Work out the finished part from the listing and answer in its coordinate system (mm). Face numbers are marked on the shaded views. Give positions to 0.01 mm unless a question says otherwise; leave off trailing zeros. Loops run counter-clockwise (first coordinate to the right, second up) from the corner with the lowest first, then second, coordinate; pieces in that order, holes last.
```python
from build123d import *

# Parameters (mm, degrees)
SKETCH2_R           = 17.416697508
BOSS_EXTRUDE1_DEPTH = 20
SKETCH7_R           = 17.416697508
CUT_EXTRUDE2_DEPTH  = 20
CIRPATTERN1_COUNT   = 6
SKETCH8_R           = 33.646475863
BOSS_EXTRUDE2_DEPTH = 30
SKETCH10_R          = 17.416697508
CUT_EXTRUDE3_DEPTH  = 30
CHAMFER1_SIZE2      = 3.639702343
CHAMFER1_SIZE       = 10


with BuildPart() as part:
    # Sketch2 → Boss-Extrude1 (new body)
    with BuildSketch(Plane.XY):
        with BuildLine():
            ThreePointArc((32.5, 121.291651246), (0, 163.646475863), (-32.5, 121.291651246))
            ThreePointArc((-32.5, 121.291651246), (-48.176762068, 83.444599647), (-88.791651246, 88.791651246))
            ThreePointArc((-88.791651246, 88.791651246), (-141.722005337, 81.823237932), (-121.291651246, 32.5))
            ThreePointArc((-121.291651246, 32.5), (-96.353524137, 0), (-121.291651246, -32.5))
            ThreePointArc((-121.291651246, -32.5), (-141.722005337, -81.823237932), (-88.791651246, -88.791651246))
            ThreePointArc((-88.791651246, -88.791651246), (-48.176762068, -83.444599647), (-32.5, -121.291651246))
            ThreePointArc((-32.5, -121.291651246), (0, -163.646475863), (32.5, -121.291651246))
            ThreePointArc((32.5, -121.291651246), (48.176762068, -83.444599647), (88.791651246, -88.791651246))
            ThreePointArc((88.791651246, -88.791651246), (141.722005337, -81.823237932), (121.291651246, -32.5))
            ThreePointArc((121.291651246, -32.5), (96.353524137, 0), (121.291651246, 32.5))
            ThreePointArc((121.291651246, 32.5), (141.722005337, 81.823237932), (88.791651246, 88.791651246))
            ThreePointArc((88.791651246, 88.791651246), (48.176762068, 83.444599647), (32.5, 121.291651246))
        make_face()
        with Locations((0, 130)):
            Circle(SKETCH2_R, mode=Mode.SUBTRACT)
        with Locations((112.583302492, 65)):
            Circle(SKETCH2_R, mode=Mode.SUBTRACT)
        with Locations((112.583302492, -65)):
            Circle(SKETCH2_R, mode=Mode.SUBTRACT)
        with Locations((0, -130)):
            Circle(SKETCH2_R, mode=Mode.SUBTRACT)
        with Locations((-112.583302492, -65)):
            Circle(SKETCH2_R, mode=Mode.SUBTRACT)
        with Locations((-112.583302492, 65)):
            Circle(SKETCH2_R, mode=Mode.SUBTRACT)
    extrude(amount=BOSS_EXTRUDE1_DEPTH)

    # Sketch4 → Revolve1 (revolve)
    with BuildSketch(Plane(origin=(0, 0, 0), x_dir=(0, 0, -1), z_dir=(1, 0, 0)), mode=Mode.PRIVATE) as revolve1_sk:
        Polygon((-20, 163.646475863), (-30, 158.646475863), (-30, 153.646475863), (-20, 153.646475863), align=None)
    revolve1 = revolve(revolve1_sk.sketch.rotate(Axis((0, 130, 0), (0, 0, 1)), 90), axis=Axis((0, 130, 0), (0, 0, 1)))

    # Sketch7 → Cut-Extrude2 (cut)
    with BuildSketch(Plane.XY):
        Circle(SKETCH7_R)
    extrude(amount=CUT_EXTRUDE2_DEPTH, mode=Mode.SUBTRACT)

    # CirPattern1: Revolve1 ×6 about axis
    cirpattern1_axis = Axis((0, 0, 0), (0, 0, 1))
    for i in range(1, CIRPATTERN1_COUNT):
        add(revolve1.rotate(cirpattern1_axis, i * 360 / CIRPATTERN1_COUNT))

    # Sketch8 → Boss-Extrude2 (add)
    with BuildSketch(Plane.XY):
        Circle(SKETCH8_R)
    extrude(amount=BOSS_EXTRUDE2_DEPTH)

    # Sketch10 → Cut-Extrude3 (cut)
    with BuildSketch(Plane.XY):
        Circle(SKETCH10_R)
    extrude(amount=CUT_EXTRUDE3_DEPTH, mode=Mode.SUBTRACT)

    # Chamfer1
    chamfer1_edges = [part.edges().sort_by_distance(p)[0] for p in [
        (-33.646475863, 0, 30),
    ]]
    chamfer1_side = [part.faces().sort_by_distance(p)[0] for p in [
        (-33.646475863, 0, 29.927205953),
    ]]
    chamfer(chamfer1_edges, length=CHAMFER1_SIZE - 0.0001, length2=CHAMFER1_SIZE2 - 0.0001, reference=chamfer1_side[0])  # a hair under: the kernel refuses the full size


solid = part.part
```
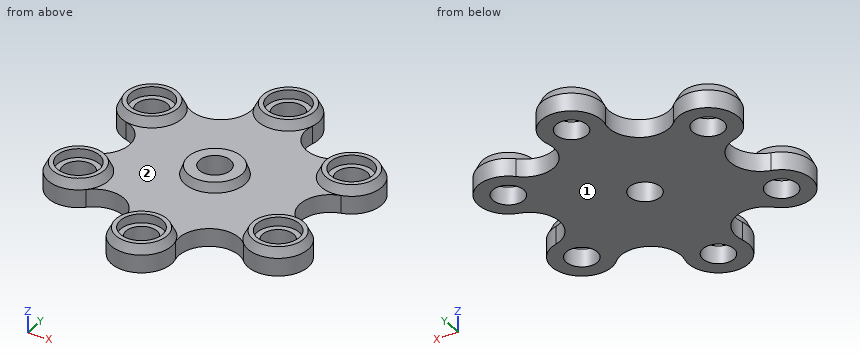
Q1. Section A-A on y = -130 is taken. Give the vertices of the cut face in (x, z).
Q2. Section D-D on x = 0 is taken. State how many separate pieces and enclosed holes the cut face has, plus the area to 3 significant figures.
Q3. Given pin 1 (10 mm diameter, centred on x = -0.5, z = 26, fed in from -Y); pin 2 (2 mm diameter, centred on x = -17.5, y = 58.5, fed in from +Z); pin 3 (12 mm diameter, centred on y = 83, z = 4, fed in from -X); pin 4 (23.5 mm diameter, centred on x = -2.5, y = 131, fed in from +Z), each flat-ended and moving along its own axis, determine where each tip first touches the part or whether it passes through.
Q4. Consider line 1 along Y through (x, z) = (110, 18.25); line 2 along Y through (x, z) = (-121.5, 27.75); line 3 along Y through (x, z) = (65, 17). Determine where each line is inside the solid, lowest interval first.
Q5. Section B-B on z = 8.5 is taken. Give the vertices of the cut face in (x, y).
Q6. Determine the mould class of the marked faces 1 and 2 for opening direction X: +X half, -X half, draft (parallel to the pull), parting line (faces both ways), or undercut.
Q7. Section C-C on y = 65 is taken. Give the vertices of the cut face in (x, z), plus the area to 3 significant figures.
Check result:
1. outline: (-33.65, 0) - (-17.42, 0) - (-17.42, 20) - (-23.65, 20) - (-23.65, 30) - (-28.65, 30) - (-33.65, 20) - close; (17.42, 0) - (33.65, 0) - (33.65, 20) - (28.65, 30) - (23.65, 30) - (23.65, 20) - (17.42, 20) - close
2. separate pieces: 4
2. enclosed holes: 0
2. area: 5,040 mm2
3. pin 1: stops at y = -163.14
3. pin 2: stops at z = 20
3. pin 3: stops at x = -144.02
3. pin 4: passes through
4. line 1: y = -98.55 to -82.22, -47.78 to -27.06, 27.06 to 47.78, 82.22 to 98.55
4. line 2: y = -93.4 to -86.9, -43.1 to -36.6, 36.6 to 43.1, 86.9 to 93.4
4. line 3: y = -78.94 to 78.94
5. outline: (-121.29, -32.5) arc R33.65 ccw (long way) to (-88.79, -88.79) arc R33.65 cw to (-32.5, -121.29) arc R33.65 ccw (long way) to (32.5, -121.29) arc R33.65 cw to (88.79, -88.79) arc R33.65 ccw (long way) to (121.29, -32.5) arc R33.65 cw to (121.29, 32.5) arc R33.65 ccw (long way) to (88.79, 88.79) arc R33.65 cw to (32.5, 121.29) arc R33.65 ccw (long way) to (-32.5, 121.29) arc R33.65 cw to (-88.79, 88.79) arc R33.65 ccw (long way) to (-121.29, 32.5) arc R33.65 cw to start; hole circle Ø34.83 at (-112.58, -65); hole circle Ø34.83 at (-112.58, 65); hole circle Ø34.83 at (0, -130); hole circle Ø34.83 at (0, 0); hole circle Ø34.83 at (0, 130); hole circle Ø34.83 at (112.58, -65); hole circle Ø34.83 at (112.58, 65)
6. face 1: draft
6. face 2: undercut
7. outline: (-146.23, 0) - (-130, 0) - (-130, 20) - (-136.23, 20) - (-136.23, 30) - (-141.23, 30) - (-146.23, 20) - close; (-95.17, 0) - (95.17, 0) - (95.17, 20) - (88.94, 20) - (88.94, 30) - (83.94, 30) - (78.94, 20) - (-78.94, 20) - (-83.94, 30) - (-88.94, 30) - (-88.94, 20) - (-95.17, 20) - close; (130, 0) - (146.23, 0) - (146.23, 20) - (141.23, 30) - (136.23, 30) - (136.23, 20) - (130, 20) - close
7. area: 4,760 mm2
